Autodesk Inventor part; units mm, degrees
ref_plane "YZ Plane" through (0, 0, 0) normal (1, 0, 0) x (0, 1, 0)
ref_plane "XZ Plane" through (0, 0, 0) normal (0, 1, 0) x (-1, 0, 0)
ref_plane "XY Plane" through (0, 0, 0) normal (0, 0, 1) x (1, 0, 0)
sketch "스케치2" plane through (0, 0, 0) normal (0, 1, 0) x (-1, 0, 0)
  line L0 (0, 0) -> (-30, 0)
  line L1 (-30, 0) -> (-30, -30)
  line L2 (-30, -30) -> (0, -30)
  line L3 (0, -30) -> (0, 0)
  line L4 (-10, -5) -> (-30, -5)
  line L5 (-30, -5) -> (-30, -25)
  line L6 (-30, -25) -> (-10, -25)
  line L7 (-10, -25) -> (-10, -5)
  point P0 (0, -15)
  point P1 (-10, -15)
  dimension "d0" = 30
  dimension "d1" = 30
  dimension "d2" = 20
  dimension "d3" = 20
extrude "돌출1" add sketch "스케치2" along normal blind 32 contours L3 L2 L1 L6 L7 L4 L0
sketch "스케치3" plane through (0, 0, -30) normal (-1, 0, 0) x (0, 0, 1)
  circle A0 centre (15, 14.6) radius 6.75
  line L0 (0, 32) -> (30, 32)
  line L1 (30, 0) -> (30, 32)
  line L2 (0, 0) -> (30, 0)
  point P0 (15, 32)
  point P1 (30, 16)
  dimension "d6" = 13.5
  dimension "d34" = 14.6
extrude "돌출2" cut sketch "스케치3" against normal blind 20
sketch "스케치4" plane through (10, 0, -5) normal (1, 0, 0) x (0, 0, -1)
  line L0 (0, 32) -> (20, 32)
  line L1 (20, 32) -> (20, 29)
  line L2 (20, 29) -> (0, 29)
  line L3 (0, 29) -> (0, 32)
  line L4 (0, 32) -> (20, 32)
  circle A0 centre (10, 14.6) radius 6.75
  line L5 (0, 0) -> (0, 32)
  point P0 (-5, 0)
  point P1 (10, 32)
  point P2 (10, 32)
  dimension "d10" = 3
  dimension "d11" = 17.4
extrude "돌출3" add sketch "스케치4" along normal up to surface (20 mm away) contours L0 L1 L2 L3
sketch "스케치6" plane through (0, 32, 0) normal (0, 1, 0) x (1, 0, 0)
  line L0 (15.85, 15) -> (69.8483, 15) construction
  line L1 (15.85, 9.15) -> (69.8483, 9.15)
  line L2 (69.8483, 20.85) -> (15.85, 20.85)
  arc A0 (15.85, 20.85) -> (15.85, 9.15) centre (15.85, 15) ccw
  arc A1 (69.8483, 9.15) -> (69.8483, 20.85) centre (69.8483, 15) ccw
  line L3 (30, 0) -> (30, 30)
  line L4 (0, 30) -> (0, 0)
  point P0 (42.8492, 15)
  point P1 (10, 15)
  point P2 (30, 15)
  point P3 (30, 9.15)
  point P4 (30, 20.85)
  dimension "d19" = 11.7
  dimension "d20" = 10
extrude "돌출5" cut sketch "스케치6" against normal blind 28 contours A0 L2 L3 L1
sketch "스케치7" plane through (10, 0, -5) normal (1, 0, 0) x (0, 0, -1)
  line L0 (0, 8) -> (20, 8)
  line L1 (20, 8) -> (20, 0)
  line L2 (20, 0) -> (0, 0)
  line L3 (0, 0) -> (0, 8)
  circle A0 centre (10, 14.6) radius 6.75
  point P0 (-5, 0)
  dimension "d32" = 8
  dimension "d33" = 8
extrude "돌출6" add sketch "스케치7" along normal up to surface (20 mm away) contours L0 A0 L1 L2 L3 | L0 A0 picked at (10.1583, 7.9556)
sketch "스케치8" plane through (30, 0, -30) normal (0, 0, -1) x (-1, 0, 0)
  line L0 (30, 0) -> (30, 32)
  line L1 (4, 17.5) -> (7, 17.5)
  line L2 (7, 17.5) -> (7, 14.5)
  line L3 (7, 14.5) -> (4, 14.5)
  line L4 (4, 14.5) -> (4, 17.5)
  point P0 (7, 16)
  point P1 (30, 16)
  dimension "d27" = 23
  dimension "d28" = 3
  dimension "d29" = 3
extrude "돌출7" cut sketch "스케치8" against normal blind 40
sketch "스케치9" plane through (30, 0, 0) normal (1, 0, 0) x (0, 0, -1)
  line L0 (0, 32) -> (9.15, 32)
  line L1 (9.15, 29) -> (9.15, 32)
  line L2 (20.85, 32) -> (20.85, 29)
  line L3 (20.85, 32) -> (30, 32)
  line L4 (9.15, 29) -> (5, 29)
  line L5 (25, 29) -> (20.85, 29)
  line L6 (0, 32) -> (0, 22)
  line L7 (0, 0) -> (0, 32)
  line L8 (30, 32) -> (30, 22)
  line L9 (0, 22) -> (5, 22)
  line L10 (5, 22) -> (5, 29)
  line L11 (25, 29) -> (25, 22)
  line L12 (25, 22) -> (30, 22)
  dimension "d35" = 10
  dimension "d36" = 10
extrude "돌출8" add sketch "스케치9" along normal blind 10
properties part number "valve_mount"
Source: CAD feature listing. Evaluate the final solid. Frame: model axes, mm. A direction names the side the tool comes from. Coordinates: 2 decimals unless noted, no trailing zeros. Loops run counter-clockwise (first coordinate to the right, second up) from the corner with the lowest first, then second, coordinate; pieces in that order, holes last. Notation, with made-up numbers: M 5.5,-2.75 L 39.5,-2.75 A9 cw 39.5,8.25 Z; hole C 82.5,88.25 d8. An arc over 180 degrees is marked long. Answer in a Markdown table with one row per item.
Q1. Section D-D on y = 4. Return the cut outline in (x, z).
Answers below:
| item | result |
|---|---|
| outline | M 0,-30 L 30,-30 L 30,0 L 0,0 Z |
Q2. Section B-B on z = -27.25. Return the cut outline in (x, y).
Answers below:
| item | result |
|---|---|
| outline | M 0,0 L 30,0 L 30,22 L 40,22 L 40,32 L 0,32 Z; hole M 23,14.5 L 26,14.5 L 26,17.5 L 23,17.5 Z |
Q3. Section C-C on y = 9.5. Return the cut outline in (x, z).
Answers below:
| item | result |
|---|---|
| outline | M 0,-30 L 30,-30 L 30,-25 L 10,-25 L 10,-19.42 L 0,-19.42 Z; M 0,-10.58 L 10,-10.58 L 10,-5 L 30,-5 L 30,0 L 0,0 Z |
Q4. Draft query along Z for faces 5 (the flat face through (25, 29, -22)), 6 (the flat face through (15, 16, 0)), 7 (the flat face through (24, 14.5, -28)). Return one class per face: pulls with the +Z half, pulls with the -Z half, needs draft (parallel to the pull), parting line crosses it, or undercut.
Answers below:
| item | result |
|---|---|
| face 5 | undercut |
| face 6 | pulls with the +Z half |
| face 7 | needs draft |
Q5. First-contact query: pin 1 (1.5 mm diameter, centred on x = 20.5, z = -10, fed in from +Y); pin 2 (12 mm diameter, centred on y = 14.6, z = -15, fed in from +X); pin 3 (6 mm diameter, centred on y = 21, z = -15.5, fed in from +X); pin 4 (1.5 mm diameter, centred on x = 37, z = -26.5, fed in from -Y). Flat tips, straight axial feed; report the tip coordinate or a pass-through.
Answers below:
| item | result |
|---|---|
| pin 1 | stops at y = 8 |
| pin 2 | passes through |
| pin 3 | stops at x = 10 |
| pin 4 | stops at y = 22 |
Q6. Section A-A on x = 31. Return the cut outline in (y, z).
Answers below:
| item | result |
|---|---|
| outline | M 22,-30 L 32,-30 L 32,-20.85 L 29,-20.85 L 29,-25 L 22,-25 Z; M 22,-5 L 29,-5 L 29,-9.15 L 32,-9.15 L 32,0 L 22,0 Z |
Q7. Ray query, probe 1 along Z at (x, y) = (6, 14.6); probe 2 along Z at (x, y) = (12, 27); probe 3 along Y at (x, z) = (3, -15). Return the intervals inside material, ascending. Write a range as from..to.
Answers below:
| item | result |
|---|---|
| probe 1 | z = -30..-21.75, -8.25..0 |
| probe 2 | z = -30..-25, -5..0 |
| probe 3 | y = 0..7.85, 21.35..32 |
Q8. Set-up query: faces 1 (the flat face through (30, 6, -15)), 2 (the flat face through (24, 14.5, -3)), 3 (the flat face through (21, 18, -5)), 4 (the flat face through (28, 31, -9.15)). Return all of +Z, -Z, +X, -X, +Y, -Y with unobstructed straight access to the full face (end or side cutting, diameter ignored); none if empty.
Answers below:
| item | result |
|---|---|
| face 1 | +Z, -Z, +X, -Y |
| face 2 | +Z, -Z |
| face 3 | +X |
| face 4 | +X, +Y |
